Geometry: see drawing. Coordinates: mm, zero at the bounding-box minimum. A direction names the side the tool comes from. Give positions to 0.01 mm unless a question says otherwise; leave off trailing zeros. Loops run counter-clockwise (first coordinate to the right, second up) from the corner with the lowest first, then second, coordinate; pieces in that order, holes last. Notation, with made-up numbers: M 54.5,-27 L 72.5,-27 A11 ccw 72.5,-13 Z; hole C -19,-38.75 d6. An arc over 180 degrees is marked long. Answer in a Markdown table with one row per item.
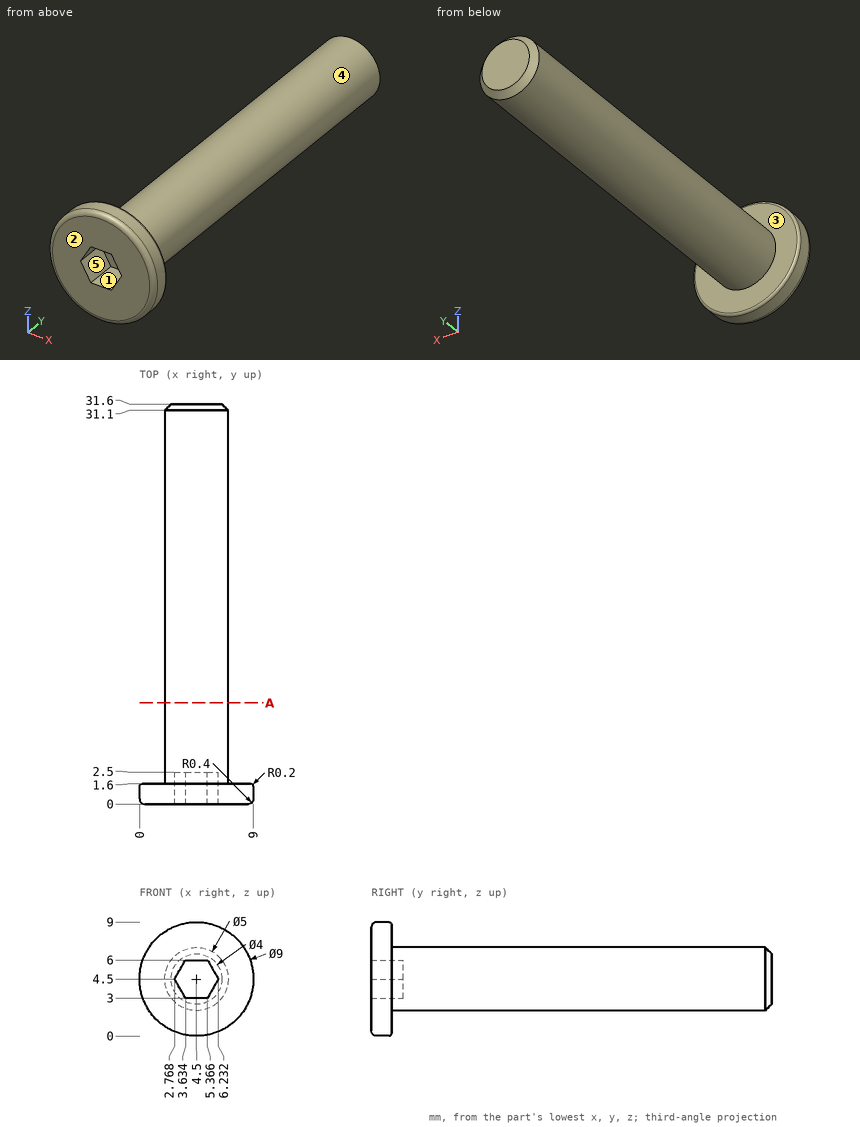
1) Pull-direction query (Z, two-part tool) for the marked faces 3, 4 and 5; classes: released by +Z, released by -Z, zero draft, split by the parting line, or undercut.
Reply:
| item | result |
|---|---|
| face 3 | zero draft |
| face 4 | split by the parting line |
| face 5 | undercut |
2) Material intervals for L1, parallel to Z at x = 4.5, y = 7.5; L2, parallel to Z at x = 2.5, y = 3; L3, parallel to Y at x = 4.25, z = 8.5, sorted ascending.
Reply:
| item | result |
|---|---|
| L1 | z = 2 to 7 |
| L2 | z = 3 to 6 |
| L3 | y = 0 to 1.6 |
3) Section A-A, the plane y = 8. Return loops of the section in (x, z), then the cut area to 3 significant figures.
Reply:
| item | result |
|---|---|
| outline | C 4.5,4.5 d5 |
| area | 19.6 mm² |
4) Set-up query: the marked faces 1 and 2. Return all of +Z, -Z, +X, -X, +Y, -Y with unobstructed straight access to the full face (end or side cutting, diameter ignored); none if empty.
Reply:
| item | result |
|---|---|
| face 1 | -Y |
| face 2 | +Z, -Z, +X, -X, -Y |
5) Pin query (flat end, axial travel): pin 1 Ø1.5 at (x, y) = (1.5, 19.5) entering from -Z; pin 2 Ø1.5 at (x, z) = (2, 1) entering from +Y. Return the tip coordinate at first contact, or that it passes through.
Reply:
| item | result |
|---|---|
| pin 1 | stops at z = 3.41 |
| pin 2 | stops at y = 1.6 |
